```python
from build123d import *

# Parameters (mm, degrees)
SKETCH1_W                  = 24.3
SKETCH1_H                  = 38
BASE_DEPTH                 = 2
SKETCH2_W                  = 24.3
SKETCH2_H                  = 38
SKETCH2_W_2                = 18.3
SKETCH2_H_2                = 31.3
PCB_EDGE_WALLS_DEPTH       = 1.7
SKETCH3_R                  = 0.95
PCB_MOUNT_DOWELS_DEPTH     = 1.6
SKETCH4_W                  = 15
SKETCH4_H                  = 15
SILICONE_PAD_HOLE_DEPTH    = 44.385510254
SKETCH6_W                  = 10.4
SKETCH6_H                  = 2.8
WIRE_SOLDERINGS_HOLE_DEPTH = 1.5
SKETCH7_W                  = 3
SKETCH7_H                  = 1.5
CUT_EXTRUDE4_DEPTH         = 1.5
SILICONE_CHANNELS_START    = -1
SKETCH5_R                  = 0.95
SKETCH5_W                  = 5
SKETCH5_H                  = 2.49
SKETCH5_W_2                = 1
SKETCH5_H_2                = 2
SILICONE_CHANNELS_DEPTH    = 1
SKETCH8_W                  = 23.48
SKETCH8_H                  = 1
CUT_EXTRUDE5_DEPTH         = 1
SKETCH9_W                  = 23.48
SKETCH9_H                  = 1
CUT_EXTRUDE6_DEPTH         = 1
FILLET1_R                  = 0.7
SKETCH17_W                 = 3
SKETCH17_H                 = 38
BOSS_EXTRUDE4_DEPTH        = 5
SKETCH19_R                 = 1.1
CUT_EXTRUDE9_DEPTH         = 5
SKETCH20_R                 = 2.1
CUT_EXTRUDE10_DEPTH        = 2
SKETCH21_R                 = 1.1
CUT_EXTRUDE11_DEPTH        = 5
SKETCH22_R                 = 2.1
CUT_EXTRUDE12_DEPTH        = 2
FILLET3_R                  = 2.5


with BuildPart() as part:
    # Sketch1 → base (new body)
    with BuildSketch(Plane(origin=(0, 0, 0), x_dir=(1, 0, 0), z_dir=(0, 1, 0))):
        with Locations((9, 18.7)):
            Rectangle(SKETCH1_W, SKETCH1_H)
    extrude(amount=BASE_DEPTH)

    # Sketch2 → pcb_edge_walls (add)
    with BuildSketch(Plane.XZ):
        with Locations((9, -18.7)):
            Rectangle(SKETCH2_W, SKETCH2_H)
        with Locations((9, -15.5)):
            Rectangle(SKETCH2_W_2, SKETCH2_H_2, mode=Mode.SUBTRACT)
    extrude(amount=PCB_EDGE_WALLS_DEPTH)

    # Sketch3 → pcb_mount_dowels (add)
    with BuildSketch(Plane.XZ):
        with Locations(Location((1.5, -29.46, 0), (0, 0, 90))):
            Circle(SKETCH3_R)
        with Locations(Location((16.5, -29.46, 0), (0, 0, 90))):
            Circle(SKETCH3_R)
        with Locations(Location((9, -3, 0), (0, 0, 90))):
            Circle(SKETCH3_R)
    extrude(amount=PCB_MOUNT_DOWELS_DEPTH)

    # Sketch4 → silicone_pad_hole (cut, through all)
    with BuildSketch(Plane(origin=(0, 2, 0), x_dir=(1, 0, 0), z_dir=(0, 1, 0))):
        with Locations((9, 12.46)):
            Rectangle(SKETCH4_W, SKETCH4_H)
    extrude(amount=-SILICONE_PAD_HOLE_DEPTH, mode=Mode.SUBTRACT)

    # Sketch6 → wire_solderings_hole (cut)
    with BuildSketch(Plane.XZ):
        with Locations((9, -26.6)):
            Rectangle(SKETCH6_W, SKETCH6_H)
    extrude(amount=-WIRE_SOLDERINGS_HOLE_DEPTH, mode=Mode.SUBTRACT)

    # Sketch7 → Cut-Extrude4 (cut)
    with BuildSketch(Plane.XZ):
        with Locations((11.7, -20.7)):
            Rectangle(SKETCH7_W, SKETCH7_H)
    extrude(amount=-CUT_EXTRUDE4_DEPTH, mode=Mode.SUBTRACT)

    # Sketch5 → silicone_channels (cut)
    with BuildSketch(Plane.XZ.offset(SILICONE_CHANNELS_START)):
        Polygon((-0.15, -19.96), (-0.15, -24.2), (18.15, -24.2), (18.15, -0.72), (-0.15, -0.72), align=None)
        with Locations(Location((9, -3, 0), (0, 0, 270))):
            Circle(SKETCH5_R, mode=Mode.SUBTRACT)
        with Locations((11.7, -21.205)):
            Rectangle(SKETCH5_W, SKETCH5_H, mode=Mode.SUBTRACT)
        Polygon((4.025, -19.96), (4.025, -21.45), (2.525, -21.45), (2.525, -22.45), (6.525, -22.45), (6.525, -21.45), (5.025, -21.45), (5.025, -19.96), align=None, mode=Mode.SUBTRACT)
        Polygon((3.858394778, -4.96), (3.858394778, -3.47), (2.358394778, -3.47), (2.358394778, -2.47), (6.358394778, -2.47), (6.358394778, -3.47), (4.858394778, -3.47), (4.858394778, -4.96), align=None, mode=Mode.SUBTRACT)
        Polygon((13.141605222, -4.96), (13.141605222, -3.47), (11.641605222, -3.47), (11.641605222, -2.47), (15.641605222, -2.47), (15.641605222, -3.47), (14.141605222, -3.47), (14.141605222, -4.96), align=None, mode=Mode.SUBTRACT)
        with Locations((1, -5.96)):
            Rectangle(SKETCH5_W_2, SKETCH5_H_2, mode=Mode.SUBTRACT)
        with Locations((1, -10.293333333)):
            Rectangle(SKETCH5_W_2, SKETCH5_H_2, mode=Mode.SUBTRACT)
        with Locations((1, -14.626666667)):
            Rectangle(SKETCH5_W_2, SKETCH5_H_2, mode=Mode.SUBTRACT)
        with Locations((1, -18.96)):
            Rectangle(SKETCH5_W_2, SKETCH5_H_2, mode=Mode.SUBTRACT)
        with Locations((17, -18.96)):
            Rectangle(SKETCH5_W_2, SKETCH5_H_2, mode=Mode.SUBTRACT)
        with Locations((17, -14.626666667)):
            Rectangle(SKETCH5_W_2, SKETCH5_H_2, mode=Mode.SUBTRACT)
        with Locations((17, -10.293333333)):
            Rectangle(SKETCH5_W_2, SKETCH5_H_2, mode=Mode.SUBTRACT)
        with Locations((17, -5.96)):
            Rectangle(SKETCH5_W_2, SKETCH5_H_2, mode=Mode.SUBTRACT)
    extrude(amount=SILICONE_CHANNELS_DEPTH, mode=Mode.SUBTRACT)

    # Sketch8 → Cut-Extrude5 (cut)
    with BuildSketch(Plane(origin=(-0.15, 0, 0), x_dir=(0, 0, -1), z_dir=(1, 0, 0))):
        with Locations((12.46, 0.5)):
            Rectangle(SKETCH8_W, SKETCH8_H)
    extrude(amount=-CUT_EXTRUDE5_DEPTH, mode=Mode.SUBTRACT)

    # Sketch9 → Cut-Extrude6 (cut)
    with BuildSketch(Plane.ZY.offset(-18.15)):
        with Locations((-12.46, 0.5)):
            Rectangle(SKETCH9_W, SKETCH9_H)
    extrude(amount=-CUT_EXTRUDE6_DEPTH, mode=Mode.SUBTRACT)

    # Fillet1
    fillet1_edges = [part.edges().sort_by_distance(p)[0] for p in [
        (-1.15, 0, -12.46),
        (19.15, 0, -12.46),
    ]]
    fillet(fillet1_edges, radius=FILLET1_R)

    # Sketch17 → Boss-Extrude4 (add)
    with BuildSketch(Plane.XZ.offset(1.7)):
        with Locations((-1.65, -18.7)):
            Rectangle(SKETCH17_W, SKETCH17_H)
        with Locations((19.65, -18.7)):
            Rectangle(SKETCH17_W, SKETCH17_H)
    extrude(amount=BOSS_EXTRUDE4_DEPTH)

    # Sketch19 → Cut-Extrude9 (cut)
    with BuildSketch(Plane.ZY.offset(3.15)):
        with Locations((-4.7, -4.2)):
            Circle(SKETCH19_R)
        with Locations((-32.7, -4.2)):
            Circle(SKETCH19_R)
    extrude(amount=-CUT_EXTRUDE9_DEPTH, mode=Mode.SUBTRACT)

    # Sketch20 → Cut-Extrude10 (cut)
    with BuildSketch(Plane.ZY.offset(3.15)):
        with Locations((-4.7, -4.2)):
            Circle(SKETCH20_R)
        with Locations((-32.7, -4.2)):
            Circle(SKETCH20_R)
    extrude(amount=-CUT_EXTRUDE10_DEPTH, mode=Mode.SUBTRACT)

    # Sketch21 → Cut-Extrude11 (cut)
    with BuildSketch(Plane(origin=(21.15, 0, 0), x_dir=(0, 0, -1), z_dir=(1, 0, 0))):
        with Locations((18.7, -4.2)):
            Circle(SKETCH21_R)
    extrude(amount=-CUT_EXTRUDE11_DEPTH, mode=Mode.SUBTRACT)

    # Sketch22 → Cut-Extrude12 (cut)
    with BuildSketch(Plane(origin=(21.15, 0, 0), x_dir=(0, 0, -1), z_dir=(1, 0, 0))):
        with Locations((18.7, -4.2)):
            Circle(SKETCH22_R)
    extrude(amount=-CUT_EXTRUDE12_DEPTH, mode=Mode.SUBTRACT)

    # Fillet3
    fillet3_edges = [part.edges().sort_by_distance(p)[0] for p in [
        (21.15, 2, -18.7),
        (-3.15, 2, -18.7),
        (21.15, -4.2, 0.3),
        (-3.15, -4.2, 0.3),
        (9, 2, 0.3),
    ]]
    fillet(fillet3_edges, radius=FILLET3_R)


solid = part.part
```
Verification items for the finished model (mm, model axes). A direction names the side the tool comes from. Round coordinates to 2 decimals unless told otherwise and drop trailing zeros. Order: outer loops, then holes, each group sorted by start corner. A loop starts at its lowest first (then second) coordinate and runs counter-clockwise, first axis right, second up. Notation, with made-up numbers: (62.25, -30) - (95.25, -30) arc R30 cw to (95.25, 7) - close; hole circle Ø7 at (35.25, 16). An arc over 180 degrees is marked (long way). Use CSV: the item, a comma, the result in double quotes. Start each with the question number.
1) Access from +Z, -Z, +X, -X, +Y, -Y to the whole of each face (thin tool, end or side, straight path). Record for faces 1 (the flat face through (-1.15, -5.1, -31.8)), 2 (the flat face through (17.5, 0.5, -14.6)).
2) Go/stop test with flat-tipped pins: P1, Ø3, axis at y = 1, z = -6, coming from the +X side; P2, Ø0.8, axis at y = 0.5, z = -22, coming from the -X side; P3, Ø0.5, axis at x = 1, z = -5.5, coming from the -Y side; P4, Ø0.5, axis at y = 0.5, z = -19.5, coming from the -X side. Record where each tip stops, or that it passes through.
3) Section check D-D, the plane z = -27.5. Record the cut outline in (x, y), plus the area to 3 significant figures.
4) Mould release check, pull along X, two halves, no side actions. Record for faces 3 (the cylindrical face through (-0.657, -4.621, -31.684)), 4 (the flat face through (19.15, -5, -20)), 5 (the flat face through (9, 0, 0)): +X half, -X half, draft (parallel to the pull), parting line (faces both ways), or undercut.
5) Section check A-A, the plane x = 7. Record the cut outline in (y, z), plus the area to 3 significant figures.
6) Thickness scan on L1, parallel to Y at x = -0.55, z = -4.7; L2, parallel to Z at x = 16.5, y = -1; L3, parallel to X at y = -2.5, z = -14. Record the ranges inside material, lowest first.
7) Section check C-C, the plane z = -32. Record the cut outline in (x, y).
8) Section check B-B, the plane y = -1. Record the cut outline in (x, z).
Answers:
1,face 1,"-X"
1,face 2,"-Y"
2,P1,"stops at x = 21.15"
2,P2,"stops at x = -3.08"
2,P3,"stops at y = 0"
2,P4,"stops at x = -3.03"
3,outline,"(-3.15, -6.7) - (-0.15, -6.7) - (-0.15, 0) - (3.8, 0) - (3.8, 1.5) - (14.2, 1.5) - (14.2, 0) - (18.15, 0) - (18.15, -6.7) - (21.15, -6.7) - (21.15, -0.5) arc R2.5 ccw to (18.65, 2) - (-0.65, 2) arc R2.5 ccw to (-3.15, -0.5) - close"
3,area,"70.5 mm²"
4,face 3,"draft"
4,face 4,"+X half"
4,face 5,"undercut"
5,outline,"(-1.7, -37.7) - (2, -37.7) - (2, -19.96) - (1, -19.96) - (1, -24.2) - (0, -24.2) - (0, -25.2) - (1.5, -25.2) - (1.5, -28) - (0, -28) - (0, -31.15) - (-1.7, -31.15) - close; (-1.7, 0.15) - (0, 0.15) - (0, -0.72) - (1, -0.72) - (1, -4.96) - (2, -4.96) - (2, -2.2) arc R2.5 ccw to (-0.5, 0.3) - (-1.7, 0.3) - close"
5,area,"43.4 mm²"
6,L1,"y = -6.7 to -5.3, -3.1 to 0.01, 1 to 2"
6,L2,"z = -37.7 to -31.15, -30.41 to -28.51, 0.15 to 0.3"
6,L3,"x = -3.15 to -0.15, 18.15 to 21.15"
7,outline,"(-3.15, -6.7) - (-0.15, -6.7) - (-0.15, -5.05) - (-1.15, -5.05) - (-1.15, -6.18) - (-3.15, -6.18) - close; (-3.15, -2.22) - (-1.15, -2.22) - (-1.15, -3.35) - (-0.15, -3.35) - (-0.15, -1.7) - (18.15, -1.7) - (18.15, -6.7) - (21.15, -6.7) - (21.15, -0.5) arc R2.5 ccw to (18.65, 2) - (-0.65, 2) arc R2.5 ccw to (-3.15, -0.5) - close"
8,outline,"(-3.15, -37.7) - (21.15, -37.7) - (21.15, -2.2) arc R2.5 ccw to (18.65, 0.3) - (-0.65, 0.3) arc R2.5 ccw to (-3.15, -2.2) - close; circle Ø1.9 at (1.5, -29.46); circle Ø1.9 at (9, -3); circle Ø1.9 at (16.5, -29.46); hole (-0.15, -31.15) - (18.15, -31.15) - (18.15, 0.15) - (-0.15, 0.15) - close"
